Could you check a few things on this model? Use its own coordinates, in mm. Face numbers are marked on the shaded views. A direction names the side the tool comes from. Round coordinates to 2 decimals unless told otherwise and drop trailing zeros. Write each loop counter-clockwise with the first axis right and the second up, starting at its lowest first coordinate (ties: lowest second). Pieces come first, ordered by that corner, then holes. Notation, with made-up numbers: M 9,78 L 42,78 A19 ccw 42,87 Z; hole C -25.75,-35 d5. An arc over 180 degrees is marked long. One line per item, written item: value. Start each with the question number.
(1) I'm going to push flat-ended pins straight in: pin 1 Ø2 at (x, y) = (1, 5) entering from +Z; pin 2 Ø1 at (x, z) = (-16, 3.5) entering from -Y; pin 3 Ø1 at (x, z) = (8, 3) entering from -Y; pin 4 Ø6 at (x, y) = (-11, 10) entering from -Z. Where does each tip first touch, or does it pass through?
(2) I want a section at D-D on x = 20.5. Please give me the cut outline in (y, z).
(3) I want a section at B-B on y = 0. Please give me the cut outline in (x, z).
(4) Which directions (+Z, -Z, +X, -X, +Y, -Y) give clear straight access to the entire face, cutting with the end or side of a thin tool? Please do the marked faces 1 and 2.
(5) Thinking about a two-plate mould opening in X: for the marked faces 3, 4, 5 and 6, which applies, released by +X, released by -X, zero draft, split by the parting line, or undercut?
(6) I want a section at A-A on z = 3.05. Please give me the cut outline in (x, y).
(7) If I drill on L1, parallel to X at y = 0, z = 2.55; L2, parallel to X at y = 44.5, z = 0.3; L3, parallel to X at y = -0.5, z = 0.5, over which ranges is the centre line in solid material (lowest first)?
(8) I want a section at C-C on y = 63.5. Please give me the cut outline in (x, z).
```python
from build123d import *

# Parameters (mm, degrees)
PAD_DEPTH    = 4
POCKET_DEPTH = 3


with BuildPart() as part:
    # Sketch → Pad (new body)
    with BuildSketch(Plane.XY):
        with BuildLine():
            Line((2.5, 18), (2.5, 48))
            ThreePointArc((15.021703, 69.663151), (5.855631, 60.510847), (2.5, 48))
            ThreePointArc((27.5, 70), (21.224622, 71.173643), (15.021703, 69.663151))
            ThreePointArc((27.5, 70), (9.351891, 70.925767), (0, 55.345233))
            ThreePointArc((0, 55.345233), (-9.351891, 70.925767), (-27.5, 70))
            ThreePointArc((-15.021703, 69.663151), (-21.224622, 71.173643), (-27.5, 70))
            ThreePointArc((-2.5, 48), (-5.855631, 60.510847), (-15.021703, 69.663151))
            Line((-2.5, 48), (-2.5, 18))
            Line((-2.5, 18), (-5.5, 15))
            Line((-5.5, 15), (-5.5, -3))
            Line((-5.5, -3), (-3.5, -5))
            Line((-3.5, -5), (3.5, -5))
            Line((3.5, -5), (5.5, -3))
            Line((5.5, -3), (5.5, 15))
            Line((5.5, 15), (2.5, 18))
        make_face()
    extrude(amount=PAD_DEPTH)

    # Sketch001 → Pocket (cut)
    with BuildSketch(Plane.XY.offset(4)):
        with BuildLine():
            ThreePointArc((-3, 2.165641), (0, -3.7), (3, 2.165641))
            Line((2.4, 13.90001), (3, 2.165641))
            ThreePointArc((2.4, 13.90001), (0, 16.3), (-2.4, 13.90001))
            Line((-3, 2.165641), (-2.4, 13.90001))
        make_face()
    extrude(amount=-POCKET_DEPTH, mode=Mode.SUBTRACT)


solid = part.part
```
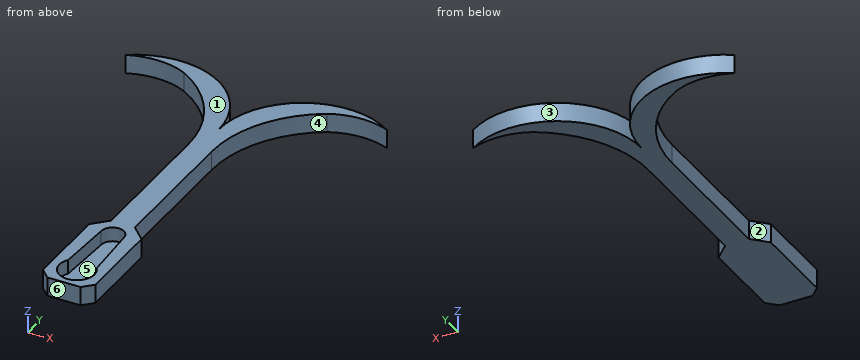
Found:
1. pin 1: stops at z = 1
1. pin 2: stops at y = 69.88
1. pin 3: stops at y = 63
1. pin 4: passes through
2. outline: M 71.14,0 L 72.77,0 L 72.77,4 L 71.14,4 Z
3. outline: M -5.5,0 L 5.5,0 L 5.5,4 L 3.7,4 L 3.7,1 L -3.7,1 L -3.7,4 L -5.5,4 Z
4. face 1: +Z, +X, -X, +Y, -Y
4. face 2: +Z, -Z, -X
5. face 3: undercut
5. face 4: released by +X
5. face 5: undercut
5. face 6: zero draft
6. outline: M -27.5,70 A15.18 cw -15.02,69.66 A25 cw -2.5,48 L -2.5,18 L -5.5,15 L -5.5,-3 L -3.5,-5 L 3.5,-5 L 5.5,-3 L 5.5,15 L 2.5,18 L 2.5,48 A25 cw 15.02,69.66 A15.18 cw 27.5,70 A17.65 ccw 0,55.35 A17.65 ccw Z; hole M -3,2.17 A3.7 ccw long 3,2.17 L 2.4,13.9 A2.4 ccw -2.4,13.9 Z
7. L1: x = -5.5 to -3.7, 3.7 to 5.5
7. L2: x = -2.5 to 2.5
7. L3: x = -5.5 to 5.5
8. outline: M -7.88,0 L -2,0 L -2,4 L -7.88,4 Z; M 2,0 L 7.88,0 L 7.88,4 L 2,4 Z
